Check sheet for the modelled part. Datum: model origin and axes. Units: mm. A direction names the side the tool comes from. Give positions to 0.01 mm unless a question says otherwise; leave off trailing zeros. Write each loop counter-clockwise with the first axis right and the second up, starting at its lowest first coordinate (ties: lowest second). Pieces come first, ordered by that corner, then holes. Notation, with made-up numbers: M 57.25,32.5 L 74.25,32.5 A22 cw 74.25,62.5 Z; hole C 47.5,74.25 d9. An arc over 180 degrees is marked long. Write each question's results on one line, items separated by ' | '. Start each with the question number.
from build123d import *

# Parameters (mm, degrees)
SKETCH1_R           = 19.15
BOSS_EXTRUDE1_DEPTH = 34.75
SKETCH2_R           = 10
BOSS_EXTRUDE2_DEPTH = 6.25
SKETCH3_R           = 3
BOSS_EXTRUDE3_DEPTH = 15
CUT_EXTRUDE1_DEPTH  = 15
SKETCH5_R           = 6.5
BOSS_EXTRUDE4_DEPTH = 25


with BuildPart() as part:
    # Sketch1 → Boss-Extrude1 (new body)
    with BuildSketch(Plane.XY):
        Circle(SKETCH1_R)
    extrude(amount=BOSS_EXTRUDE1_DEPTH)

    # Sketch2 → Boss-Extrude2 (add)
    with BuildSketch(Plane.XY.offset(34.75)):
        Circle(SKETCH2_R)
    extrude(amount=BOSS_EXTRUDE2_DEPTH)

    # Sketch3 → Boss-Extrude3 (add)
    with BuildSketch(Plane.XY.offset(41)):
        Circle(SKETCH3_R)
    extrude(amount=BOSS_EXTRUDE3_DEPTH)

    # Sketch4 → Cut-Extrude1 (cut)
    with BuildSketch(Plane.XY.offset(56)):
        with BuildLine():
            Line((-1.658312395, 2.5), (1.658312395, 2.5))
            ThreePointArc((1.658312395, 2.5), (0, 3), (-1.658312395, 2.5))
        make_face()
    extrude(amount=-CUT_EXTRUDE1_DEPTH, mode=Mode.SUBTRACT)

    # Sketch5 → Boss-Extrude4 (add)
    with BuildSketch(Plane(origin=(0, 0, 0), x_dir=(1, 0, 0), z_dir=(0, 1, 0))):
        with Locations((0, -6.5)):
            Circle(SKETCH5_R)
    extrude(amount=BOSS_EXTRUDE4_DEPTH)


solid = part.part
Q1. Section check B-B on z = 31.5. Record the boundary of the cut face in (x, y), plus the area to 3 significant figures.
Q2. Tool access check on faces 1 (the face through (2.999, 21.458, 12.267)), 2 (the face through (0, 2.5, 49)), 3 (the face through (0, -3, 48)). Record the directions out of +Z, -Z, +X, -X, +Y, -Y that give a thin tool (end or side, any length) a straight path to the whole face; none if there is none.
Q3. Section check D-D on y = -5. Record the boundary of the cut face in (x, z), plus the area to 3 significant figures.
Q4. Scan lines: L1, parallel to Y at x = 0.5, z = 17; L2, parallel to Z at x = -13, y = -1; L3, parallel to Z at x = -3, y = 3.5. Record each from-to range of solid material in increasing order.
Q5. Depth check by flat-ended pin: pin 1 Ø5 at (y, z) = (-2.5, 44) entering from +X; pin 2 Ø5 at (y, z) = (19, 9.5) entering from +X; pin 3 Ø3 at (x, y) = (3.5, 18) entering from +Z. Enter the tip coordinate at first touch or a pass-through.
Q6. Section check A-A on y = 0. Record the boundary of the cut face in (x, z).
Q7. Section check C-C on x = 12. Record the boundary of the cut face in (y, z), plus the area to 3 significant figures.
Check result:
1) outline: C 0,0 d38.3 | area: 1,150 mm^2
2) face 1: +Y | face 2: +Z, +X, -X, +Y | face 3: +Z
3) outline: M -18.49,0 L 18.49,0 L 18.49,34.75 L 8.66,34.75 L 8.66,41 L -8.66,41 L -8.66,34.75 L -18.49,34.75 Z | area: 1,390 mm^2
4) L1: -19.14 to 19.14 | L2: 0 to 34.75 | L3: 0 to 41
5) pin 1: x = 3 | pin 2: x = 9.72 | pin 3: z = 34.75
6) outline: M -19.15,0 L 19.15,0 L 19.15,34.75 L 10,34.75 L 10,41 L 3,41 L 3,56 L -3,56 L -3,41 L -10,41 L -10,34.75 L -19.15,34.75 Z
7) outline: M -14.92,0 L 14.92,0 L 14.92,34.75 L -14.92,34.75 Z | area: 1,040 mm^2
